Geometry check sheet. Reference: the model listing, model coordinates, mm. Round coordinates to 2 decimals unless told otherwise and drop trailing zeros. Order: outer loops, then holes, each group sorted by start corner. A loop starts at its lowest first (then second) coordinate and runs counter-clockwise, first axis right, second up.
(1) Go/stop test with flat-tipped pins: pin 1 (2.5 mm diameter, centred on y = 1, z = 5.5, fed in from +X); pin 2 (3.5 mm diameter, centred on x = 63, y = 0, fed in from +Z); pin 3 (2.5 mm diameter, centred on x = -64, y = -0.5, fed in from +Z); pin 4 (2 mm diameter, centred on y = -1, z = 4.5, fed in from -X). Record where each tip stops, or that it passes through.
(2) Material ranges on line 1 along Y through (x, z) = (-64, 1.2); line 2 along X through (y, z) = (0.5, 1.25); line 3 along X through (y, z) = (3.5, 5.5), recorded low to high.
(3) Sectioned sample at C-C (x = 48). Record the boundary of the cut face in (y, z), plus the area to 3 significant figures.
(4) Sectioned sample at D-D (x = 33). Record the boundary of the cut face in (y, z), plus the area to 3 significant figures.
(5) Sectioned sample at B-B (z = 5.75). Record the boundary of the cut face in (x, y).
(6) Release check for a two-part mould opening along X. For faces 1 (the face through (59, -1, 4)), 2 (the face through (-59, 0, 4)), 3 (the face through (1, -7, 4)), 4 (the face through (65.43, -0.95, 0.99)) record: +X half, -X half, draft (parallel to the pull), parting line (faces both ways), or undercut.
(7) Sectioned sample at A-A (y = -0.5). Record the boundary of the cut face in (x, z), plus the area to 3 significant figures.
Autodesk Inventor part; units mm, degrees
ref_plane "YZ Plane" through (0, 0, 0) normal (1, 0, 0) x (0, 1, 0)
ref_plane "XZ Plane" through (0, 0, 0) normal (0, 1, 0) x (-1, 0, 0)
ref_plane "XY Plane" through (0, 0, 0) normal (0, 0, 1) x (1, 0, 0)
sketch "Base" plane through (0, 0, 0) normal (0, 0, 1) x (1, 0, 0)
  line L0 (-64, -0.5) -> (64, -0.5) construction
  circle A0 centre (-64, -0.5) radius 1.5
  circle A1 centre (64, -0.5) radius 1.5
  line L1 (-64, 6) -> (64, 6)
  line L2 (69, 1) -> (69, -2)
  line L3 (64, -7) -> (-64, -7)
  line L4 (-69, -2) -> (-69, 1)
  line L5 (-59, 6) -> (-59, -7) construction
  line L6 (59, 6) -> (59, -7) construction
  arc A2 (-64, 6) -> (-69, 1) centre (-64, 1) ccw
  arc A3 (-69, -2) -> (-64, -7) centre (-64, -2) ccw
  arc A4 (69, 1) -> (64, 6) centre (64, 1) ccw
  arc A5 (64, -7) -> (69, -2) centre (64, -2) ccw
  point P0 (0, 0)
  dimension "d0" = 128
  dimension "d1" = 3
  dimension "d2" = 3
  dimension "d3" = 5
  dimension "d4" = 5
  dimension "d5" = 5
  dimension "d6" = 5
  dimension "d7" = 5
  dimension "d8" = 6.5
  dimension "d9" = 6.5
extrude "BaseFeature" add sketch "Base" along normal blind 2
sketch "Sketch2" plane through (0, 0, 2) normal (0, 0, 1) x (1, 0, 0)
  line L0 (-59, 6) -> (-59, -7) construction
  line L1 (59, 6) -> (59, -7) construction
  line L2 (58, 6) -> (-58, 6)
  line L3 (64, 6) -> (-64, 6) construction
  line L4 (-59, 5) -> (-59, -6)
  line L5 (-58, -7) -> (58, -7)
  line L6 (59, -6) -> (59, 5)
  arc A0 (-58, 6) -> (-59, 5) centre (-58, 5) ccw
  arc A1 (-59, -6) -> (-58, -7) centre (-58, -6) ccw
  arc A2 (59, 5) -> (58, 6) centre (58, 5) ccw
  arc A3 (58, -7) -> (59, -6) centre (58, -6) ccw
  point P0 (0, 0)
  dimension "d12" = 1
  dimension "d13" = 1
extrude "Extrusion2" add sketch "Sketch2" along normal blind 6
sketch "Sketch3" plane through (-64, -7, 0) normal (0, -1, 0) x (1, 0, 0)
  line L0 (0, 0) -> (128, 0) construction
  line L1 (128, 0) -> (128, 2) construction
  line L2 (122, 2) -> (128, 2) construction
  line L3 (6, 8) -> (122, 8) construction
  line L4 (0, 2) -> (6, 2) construction
  line L5 (0, 0) -> (0, 2) construction
  line L6 (64, 0) -> (64, 8.0447) construction
  line L7 (6, 8) -> (122, 8) construction
  arc A0 (64, 8.0447) -> (5, 7) centre (53.5583, -1068.8352) ccw
  arc A1 (123, 7) -> (64, 8.0447) centre (74.4417, -1068.8352) ccw
  line L8 (5, 2) -> (5, 8)
  line L9 (123, 2) -> (123, 8)
  line L10 (123, 8) -> (5, 8)
  point P0 (88.7678, 8)
  point P1 (39.2322, 8)
  dimension "d17" = 1076.9305
  dimension "d22" = 1
  dimension "d23" = 1
extrude "Extrusion4" cut sketch "Sketch3" against normal through all contours L10 L9 A1 | A0 L8 L10
equation "\"d9\" = d8"
properties part number "MidiPickup"
Answer below:
1. pin 1: stops at x = 59
1. pin 2: stops at z = 2
1. pin 3: passes through
1. pin 4: stops at x = -59
2. line 1: y = -7 to -2, 1 to 6
2. line 2: x = -69 to -65.12, -62.88 to 62.88, 65.12 to 69
2. line 3: x = -59 to 59
3. outline: (-7, 0) - (6, 0) - (6, 7.44) - (-7, 7.44) - close
3. area: 96.7 mm2
4. outline: (-7, 0) - (6, 0) - (6, 7.86) - (-7, 7.86) - close
4. area: 102 mm2
5. outline: (-59, -6) arc R1 ccw to (-58, -7) - (58, -7) arc R1 ccw to (59, -6) - (59, 5) arc R1 ccw to (58, 6) - (-58, 6) arc R1 ccw to (-59, 5) - close
6. face 1: +X half
6. face 2: -X half
6. face 3: draft
6. face 4: undercut
7. outline: (-69, 0) - (-65.5, 0) - (-65.5, 2) - (-69, 2) - close; (-62.5, 0) - (62.5, 0) - (62.5, 2) - (59, 2) - (59, 7) arc R1076.97 ccw to (24.77, 8) - (-24.77, 8) arc R1076.89 ccw to (-59, 7) - (-59, 2) - (-62.5, 2) - close; (65.5, 0) - (69, 0) - (69, 2) - (65.5, 2) - close
7. area: 944 mm2
